```python
from build123d import *

# Parameters (mm, degrees)
F1_DEPTH = 76.2
F2_R     = 19.05
F3_DEPTH = 25.4
F4_R     = 10.16
F5_DEPTH = 101.6


with BuildPart() as f1:
    # F0 (on Front) → F1 (new body)
    with BuildSketch(Plane.XZ):
        Polygon((-38.1, 10.208864), (-38.1, -10.208864), (-27.891136, -27.891136), (-10.208864, -38.1), (10.208864, -38.1), (27.891136, -27.891136), (38.1, -10.208864), (38.1, 10.208864), (27.891136, 27.891136), (10.208864, 38.1), (-10.208864, 38.1), (-27.891136, 27.891136), align=None)
    extrude(amount=-F1_DEPTH)

    # F2 (on Front) → F3 (join)
    with BuildSketch(Plane.XZ):
        Circle(F2_R)
    extrude(amount=F3_DEPTH)

    # F4 (on face) → F5 (cut)
    with BuildSketch(Plane.XZ.offset(25.4)):
        Circle(F4_R)
    extrude(amount=-F5_DEPTH, mode=Mode.SUBTRACT)

    # F6 (on Right) → F7 (revolve, cut)
    with BuildSketch(Plane.YZ):
        Polygon((-25.4, 16.51), (-25.4, 0), (36.216159, 0), align=None)
    revolve(axis=Axis((0, 5.408079, 0), (0, -1, 0)), mode=Mode.SUBTRACT)


solid = f1.part
```
Geometry: final body of the model. Coordinates: model frame, mm. A direction names the side the tool comes from. Give positions to 0.01 mm unless a question says otherwise; leave off trailing zeros. Write each loop counter-clockwise with the first axis right and the second up, starting at its lowest first coordinate (ties: lowest second). Pieces come first, ordered by that corner, then holes.
1. Line query: probe 1 along X at (y, z) = (15.5, 0); probe 2 along Y at (x, z) = (-34, -5.5). Output: solid intervals per line, ascending.
2. Section query D-D, the plane z = 26. Return loops of the section in (x, y), then the cut area to 3 significant figures.
3. Section query B-B, the plane y = 16. Return loops of the section in (x, z), then the cut area to 3 significant figures.
4. Reachability of faces 1 (the flat face through (7.9, 0, 17.5)), 2 (the flat face through (-18.926, 37.567, 33.067)) from +Z, -Z, +X, -X, +Y, -Y: full face, straight path, thin tool, end or side. Return the list, or none.
5. Section query A-A, the plane x = 0. Return loops of the section in (y, z).
6. Section query C-C, the plane z = 0. Return loops of the section in (x, y), then the cut area to 3 significant figures.
7. Pin query (flat end, axial travel): P1, Ø2, axis at y = 45.5, z = -25.5, coming from the +X side; P2, Ø4, axis at x = 16, y = 59.5, coming from the -Z side; P3, Ø1.5, axis at x = -27, y = 60.5, coming from the +Z side. Return the tip coordinate at first contact, or that it passes through.
8. Draft query along X for faces 3 (the conical face through (12.37, -11.08, -2.75)), 4 (the cylindrical face through (-1.323, 36.704, 10.074)), 5 (the cylindrical face through (-15.12, -12.52, -11.59)), 6 (the flat face through (19.174, 37.567, 32.924)). Return one class per face: released by +X, released by -X, zero draft, split by the parting line, or undercut.
Computed:
1. probe 1: x = -38.1 to -10.16, 10.16 to 38.1
1. probe 2: y = 0 to 76.2
2. outline: (-28.98, 0) - (28.98, 0) - (28.98, 76.2) - (-28.98, 76.2) - close
2. area: 4,420 mm2
3. outline: (-38.1, -10.21) - (-27.89, -27.89) - (-10.21, -38.1) - (10.21, -38.1) - (27.89, -27.89) - (38.1, -10.21) - (38.1, 10.21) - (27.89, 27.89) - (10.21, 38.1) - (-10.21, 38.1) - (-27.89, 27.89) - (-38.1, 10.21) - close; hole circle Ø20.32 at (0, 0)
3. area: 4,340 mm2
4. face 1: -Y
4. face 2: +Z, -X, +Y, -Y
5. outline: (-25.4, -19.05) - (0, -19.05) - (0, -38.1) - (76.2, -38.1) - (76.2, -10.16) - (-1.7, -10.16) - (-25.4, -16.51) - close; (-25.4, 16.51) - (-1.7, 10.16) - (76.2, 10.16) - (76.2, 38.1) - (0, 38.1) - (0, 19.05) - (-25.4, 19.05) - close
6. outline: (-38.1, 0) - (-19.05, 0) - (-19.05, -25.4) - (-16.51, -25.4) - (-10.16, -1.7) - (-10.16, 76.2) - (-38.1, 76.2) - close; (10.16, -1.7) - (16.51, -25.4) - (19.05, -25.4) - (19.05, 0) - (38.1, 0) - (38.1, 76.2) - (10.16, 76.2) - close
6. area: 4,560 mm2
7. P1: stops at x = 29.85
7. P2: stops at z = -35.91
7. P3: stops at z = 28.84
8. face 3: undercut
8. face 4: undercut
8. face 5: split by the parting line
8. face 6: released by +X
